from build123d import *

# Parameters (mm, degrees)
SKETCH5_W           = 12
SKETCH5_H           = 16.095925532
SKETCH10_R          = 12.5
BOSS_EXTRUDE3_DEPTH = 52
SKETCH11_R          = 12.5
CUT_EXTRUDE3_DEPTH  = 109
SCALE1_SCALE        = 1.9329
SKETCH13_R          = 24.16125
BOSS_EXTRUDE4_DEPTH = 5
FILLET1_R           = 10
FILLET2_R           = 10
FILLET4_R           = 5
SCALE2_SCALE        = 1.5
SKETCH15_R          = 36.241875
BOSS_EXTRUDE5_DEPTH = 60


with BuildPart() as part:
    # Sketch1 → Revolve1 (revolve)
    with BuildSketch(Plane(origin=(0, 0, 0), x_dir=(1, 0, 0), z_dir=(0, 1, 0))):
        Polygon((-97.333333333, 12.5), (-57.433333333, 12.5), (-57.433333333, 19.5), (-55.433333333, 19.5), (-39.766666667, 7.5), (-36.533333333, 16), (-34.533333333, 16), (-34.533333333, 7.5), (-22.533333333, 7.5), (-22.533333333, 16), (-20.533333333, 16), (-18.590278059, 7.5), (5.366666667, 7.5), (5.366666667, 0), (-97.333333333, 0), align=None)
    revolve(axis=Axis((99.666666667, 0, 0), (-1, 0, 0)))

    # Sketch2 → Revolve2 (revolve)
    with BuildSketch(Plane.XY, mode=Mode.PRIVATE) as revolve2_sk:
        Polygon((5.366666667, 0), (80.644631229, 0), (80.644631229, 8.695124825), (66.612224209, 8.695124825), (55.795033147, 23.11804624), (52.466666667, 23.11804624), (52.466666667, 12.5), (5.366666667, 12.5), align=None)
    revolve(revolve2_sk.sketch.rotate(Axis((5.366666667, 0, 0), (1, 0, 0)), 90), axis=Axis((5.366666667, 0, 0), (1, 0, 0)))

    # Sketch3 → Cut-Revolve1 (revolve, cut)
    with BuildSketch(Plane.XY, mode=Mode.PRIVATE) as cut_revolve1_sk:
        Polygon((-1.866722484, 7.5), (24.866666667, 7.5), (24.866666667, 12.5), (24.866666667, 26.008660159), (-1.866722484, 26.008660159), align=None)
    revolve(cut_revolve1_sk.sketch.rotate(Axis((-112.967867012, 0, 0), (1, 0, 0)), 270), axis=Axis((-112.967867012, 0, 0), (1, 0, 0)), mode=Mode.SUBTRACT)

    # Sketch4 → Revolve3 (revolve)
    with BuildSketch(Plane.XY, mode=Mode.PRIVATE) as revolve3_sk:
        Polygon((22.366666667, 0), (22.366666667, 12.5), (20.366666667, 12.5), (17.366666667, 0), align=None)
    revolve(revolve3_sk.sketch.rotate(Axis((17.366666667, 0, 0), (1, 0, 0)), 270), axis=Axis((17.366666667, 0, 0), (1, 0, 0)))

    # Sketch5 → Cut-Revolve2 (revolve, cut)
    with BuildSketch(Plane.XY, mode=Mode.PRIVATE) as cut_revolve2_sk:
        with Locations((28.366666667, 13.047962766)):
            Rectangle(SKETCH5_W, SKETCH5_H)
    revolve(cut_revolve2_sk.sketch.rotate(Axis((-109.042031517, 0, 0), (1, 0, 0)), 90), axis=Axis((-109.042031517, 0, 0), (1, 0, 0)), mode=Mode.SUBTRACT)

    # Sketch10 → Boss-Extrude3 (add)
    with BuildSketch(Plane.ZY.offset(-34.366666667)):
        with Locations(Location((0, 0, 0), (0, 0, 180))):
            Circle(SKETCH10_R)
    extrude(amount=-BOSS_EXTRUDE3_DEPTH)

    # Sketch11 → Cut-Extrude3 (cut)
    with BuildSketch(Plane(origin=(22.366666667, 0, 0), x_dir=(0, 0, -1), z_dir=(1, 0, 0))):
        Circle(SKETCH11_R)
    extrude(amount=CUT_EXTRUDE3_DEPTH, mode=Mode.SUBTRACT)


with BuildPart() as body_2:
    # of the pieces the cut leaves, the one that is kept (cut_extrude3_keep)
    add(part.part.solids().sort_by_distance((22.366666667, 0, -12.5))[0])

    # Sketch12 → Revolve6 (revolve)
    with BuildSketch(Plane.XY, mode=Mode.PRIVATE) as revolve6_sk:
        Polygon((22.366666667, 5), (34.366666667, 5), (34.366666667, 12.5), (36.366666667, 12.5), (37.912349785, 5), (45.066666667, 19.558173299), (47.066666667, 19.558173299), (47.066666667, 15), (69.466666667, 15), (69.466666667, 19.558173299), (71.466666667, 19.558173299), (72.406065536, 15), (82.356461942, 15), (82.356461942, 0), (22.366666667, 0), align=None)
    revolve(revolve6_sk.sketch.rotate(Axis((22.366666667, 0, 0), (1, 0, 0)), 90), axis=Axis((22.366666667, 0, 0), (1, 0, 0)))


with BuildPart() as body_2_1:
    # Scale1: scaled about (-3.323692934, 0, 0)
    add(body_2.part.scale(SCALE1_SCALE).moved(Location((3.100673138, 0, 0))))

    # Sketch13 → Boss-Extrude4 (add)
    with BuildSketch(Plane.ZY.offset(185.034926862)):
        with Locations(Location((0, 0, 0), (0, 0, 180))):
            Circle(SKETCH13_R)
    extrude(amount=BOSS_EXTRUDE4_DEPTH)

    # Fillet1
    fillet1_edges = [body_2_1.edges().sort_by_distance(p)[0] for p in [
        (-73.764316862, 0, 14.49675),
    ]]
    fillet(fillet1_edges, radius=FILLET1_R)

    # Fillet2
    # the kernel refuses this fillet: 10 mm, written as the material it adds along each edge
    with BuildSketch(Plane(origin=(40.147923138, 0, 0), x_dir=(0, 0, -1), z_dir=(0, -1, 0))) as fillet2_piece_1:
        with BuildLine():
            CenterArc((14.49675 + FILLET2_R, -FILLET2_R * 0.788396810575), FILLET2_R, 103.495733281, 76.504266719)
            Line((14.49675 + FILLET2_R * 0.766627047525, FILLET2_R * 0.183990491406), (14.49675 + FILLET2_R * 0.761959588475, FILLET2_R * 0.203438237446))
            Line((14.49675 + FILLET2_R * 0.761959588475, FILLET2_R * 0.203438237446), (14.49675 - FILLET2_R * 0.02, FILLET2_R * 0.0157679362115))
            Line((14.49675 - FILLET2_R * 0.02, FILLET2_R * 0.0157679362115), (14.49675 - FILLET2_R * 0.02, -FILLET2_R * 0.788396810575))
            Line((14.49675 - FILLET2_R * 0.02, -FILLET2_R * 0.788396810575), (14.49675, -FILLET2_R * 0.788396810575))
        make_face()
    revolve(axis=Axis((40.147923138, 0, 0), (1, 0, 0)))
    with BuildSketch(Plane(origin=(76.381454038, 0, 0), x_dir=(0, 0, 1), z_dir=(0, 1, 0))) as fillet2_piece_2:
        with BuildLine():
            CenterArc((33.505516614, 0.573905142), FILLET2_R, 116.170866586, 84.693418733)
            Line((29.095020982, 9.548732621), (29.00681107, 9.728229171))
            Line((29.00681107, 9.728229171), (9.576290087, 0.17949655))
            Line((9.576290087, 0.17949655), (9.624130193, -0.195883329))
            ThreePointArc((9.624130193, -0.195883329), (16.872505193, -1.689708779), (23.974364668, -3.058882021))
            Line((23.974364668, -3.058882021), (24.16125, -2.9876509))
        make_face()
    revolve(axis=Axis((76.381454038, 0, 0), (1, 0, 0)))
    with BuildSketch(Plane(origin=(-32.832475321, 0, 0), x_dir=(0, 0, -1), z_dir=(0, 1, 0))) as fillet2_piece_3:
        with BuildLine():
            CenterArc((14.49675 + FILLET2_R, -FILLET2_R * 0.79720034578), FILLET2_R, 102.876270786, 77.123729214)
            Line((14.49675, -FILLET2_R * 0.79720034578), (14.49675 - FILLET2_R * 0.02, -FILLET2_R * 0.79720034578))
            Line((14.49675 - FILLET2_R * 0.02, -FILLET2_R * 0.79720034578), (14.49675 - FILLET2_R * 0.02, FILLET2_R * 0.0159440069156))
            Line((14.49675 - FILLET2_R * 0.02, FILLET2_R * 0.0159440069156), (14.49675 + FILLET2_R * 0.772696675376, FILLET2_R * 0.197150295903))
            Line((14.49675 + FILLET2_R * 0.772696675376, FILLET2_R * 0.197150295903), (14.49675 + FILLET2_R * 0.777153603309, FILLET2_R * 0.177653224497))
        make_face()
    revolve(axis=Axis((-32.832475321, 0, 0), (-1, 0, 0)))

    # Sketch14 → Revolve7 (revolve)
    with BuildSketch(Plane.XY, mode=Mode.PRIVATE) as revolve7_sk:
        Polygon((90.210033138, 0), (90.210033138, 40.883707347), (88.684603111, 40.883707347), (81.69733558, 9.377482841), (81.69733558, 0), align=None)
    revolve(revolve7_sk.sketch.rotate(Axis((81.69733558, 0, 0), (1, 0, 0)), 90), axis=Axis((81.69733558, 0, 0), (1, 0, 0)))

    # Fillet3: read off the stored shape, not the designer's step
    # Fillet3 outline → Fillet3 (revolve)
    with BuildSketch(Plane.YX):
        with BuildLine():
            Line((29.614165238, 86.185309499), (29.095020982, 85.930186659))
            ThreePointArc((29.095020982, 85.930186659), (29.874355922, 86.207955574), (30.673985231, 86.420350223))
            Line((30.673985231, 86.420350223), (29.614165238, 86.420350223))
            Line((29.614165238, 86.420350223), (29.614165238, 86.185309499))
        make_face()
    revolve(axis=Axis((0, 0, 0), (1, 0, 0)))

    # Fillet4
    # the kernel refuses this fillet: 5 mm, written as the material it adds along each edge
    with BuildSketch(Plane(origin=(85.930186659, 0, 0), x_dir=(0, 1, 0), z_dir=(0, 0, -1))) as fillet4_piece_1:
        with BuildLine():
            CenterArc((31.137752518, -4.571000373), FILLET4_R, 109.893555323, 8.371610668)
            ThreePointArc((29.4363836, 0.130631663), (29.265105411, 0.066875579), (29.095020982, 0))
            ThreePointArc((29.095020982, 0), (28.931740857, -0.082101501), (28.769988422, -0.167173266))
        make_face()
    fillet4_piece_1_solid = revolve(axis=Axis((85.930186659, 0, 0), (1, 0, 0)), revolution_arc=90, mode=Mode.PRIVATE)
    with BuildSketch(Plane(origin=(85.930186659, 0, 0), x_dir=(0, 0, 1), z_dir=(0, 1, 0))) as fillet4_piece_2:
        with BuildLine():
            CenterArc((31.137752518, -4.571000373), FILLET4_R, 109.893555323, 8.371610668)
            ThreePointArc((29.4363836, 0.130631663), (29.265105411, 0.066875579), (29.095020982, 0))
            ThreePointArc((29.095020982, 0), (28.931740857, -0.082101501), (28.769988422, -0.167173266))
        make_face()
    fillet4_piece_2_solid = revolve(axis=Axis((85.930186659, 0, 0), (1, 0, 0)), revolution_arc=270, mode=Mode.PRIVATE)
    add([fillet4_piece_1_solid, fillet4_piece_2_solid])


with BuildPart() as body_2_2:
    # Scale2: scaled about (-4.900577652, 0, 5.1e-08)
    add(body_2_1.part.scale(SCALE2_SCALE).moved(Location((2.450288826, 0, -2.6e-08))))

    # Sketch15 → Boss-Extrude5 (add)
    with BuildSketch(Plane.ZY.offset(282.602101447)):
        with Locations(Location((0, 0, 0), (0, 0, 180))):
            Circle(SKETCH15_R)
    extrude(amount=BOSS_EXTRUDE5_DEPTH)


solid = body_2_2.part
For this review, take the finished solid that the model builds, in its own axes (mm). A direction names the side the tool comes from. Round coordinates to 2 decimals unless told otherwise and drop trailing zeros. Loops run counter-clockwise (first coordinate to the right, second up) from the corner with the lowest first, then second, coordinate; pieces in that order, holes last. Notation, with made-up numbers: (-31, 76.25) - (24, 76.25) arc R34 cw to (24, 110.25) - close; hole circle Ø6 at (77, 75). An arc over 180 degrees is marked (long way). Use one line per item in the form item = value.
1) Wall thickness on probe 1 along X at (y, z) = (18.5, 44); probe 2 along X at (y, z) = (50, 4); probe 3 along X at (y, z) = (8.5, 41.5): over which ranges is each line inside the solid? List them lowest first.
Solutions:
probe_1 = -159.42 to -142.12, 132.46 to 143.56, 208.51 to 216.16
probe_2 = -159.42 to -145.29, 133 to 143.56, 208.51 to 215.66
probe_3 = -159.42 to -135.11, -100.35 to -93.02, -58.23 to -51.51, 130.64 to 245.88
2) Mouldability with a two-part tool opening along X and no side actions: class faces 4 (the face through (-159.418, 37, -1)), 5 (the face through (132.246, -14.044, 44.596)), 6 (the face through (245.882, -1, -1)), 7 (the face through (211.45, -17.03, 54.09)) as pulls with the +X half, pulls with the -X half, needs draft (parallel to the pull), parting line crosses it, or undercut.
Solutions:
face_4 = pulls with the -X half
face_5 = undercut
face_6 = pulls with the +X half
face_7 = needs draft
3) Tool access review of faces 1 (the face through (106.742, -1, -16)), 2 (the face through (216.9, 26.85, -35.02)), 3 (the face through (-156.48, 55.19, 12.26)): name each direction out of +Z, -Z, +X, -X, +Y, -Y from which nothing blocks a thin tool from reaching the whole face with its end or side.
Solutions:
face_1 = none
face_2 = +X
face_3 = -X
4) We need section A-A on x = -16.5. Write out the cut boundary in (y, z), then the cut area to 3 significant figures.
Solutions:
outline = circle Ø43.49 at (0, 0)
area = 1,490 mm2
5) Clearance check with flat-ended pins moving along their axes: P1, Ø2, axis at x = -236.5, y = 32.5, coming from the +Z side; P2, Ø1, axis at x = -153, z = 26.5, coming from the +Y side. State where each tip first meets the part, or that it passes through.
Solutions:
P1 = 17.92
P2 = 49.91
